Geometry: final body of the model. Coordinates: model frame, mm. Give positions to 0.01 mm unless a question says otherwise; leave off trailing zeros. Loops run counter-clockwise (first coordinate to the right, second up) from the corner with the lowest first, then second, coordinate; pieces in that order, holes last.
1. First-contact query: P1, Ø0.8, axis at y = 33.5, z = 0.5, coming from the -X side; P2, Ø0.8, axis at y = 17.5, z = 1, coming from the -X side. Flat tips, straight axial feed; report the tip coordinate or a pass-through.
2. Section A-A, the plane y = 32.5. Output: boundary loops of the cut face in (x, z), then the cut area to 3 significant figures.
3. Section C-C, the plane y = 7.1. Output: boundary loops of the cut face in (x, z), then the cut area to 3 significant figures.
4. Section D-D, the plane z = 0.9. State how many separate pieces and enclosed holes the cut face has, then the cut area to 3 significant figures.
5. Material intervals for line 1 along Y through (x, z) = (2, 0.65); line 2 along X through (y, z) = (60.5, 0.85); line 3 along Y through (x, z) = (13, 0.2), sorted ascending.
6. Section B-B, the plane x = 11.6. Output: boundary loops of the cut face in (y, z), then the cut area to 3 significant figures.
Autodesk Inventor part; units mm, degrees
ref_plane "YZ Plane" through (0, 0, 0) normal (1, 0, 0) x (0, 1, 0)
ref_plane "XZ Plane" through (0, 0, 0) normal (0, 1, 0) x (-1, 0, 0)
ref_plane "XY Plane" through (0, 0, 0) normal (0, 0, 1) x (1, 0, 0)
sketch "スケッチ1" plane through (0, 0, 0) normal (0, 0, 1) x (1, 0, 0)
  line L0 (0, 0) -> (32, 0)
  line L1 (32, 0) -> (32, 63)
  line L2 (32, 63) -> (0, 63)
  line L3 (0, 63) -> (0, 0)
  dimension "d0" = 32
  dimension "d1" = 63
extrude "押し出し1" add sketch "スケッチ1" along normal blind 1.5
sketch "スケッチ2" plane through (0, 0, 1.5) normal (0, 0, 1) x (1, 0, 0)
  line L0 (2, 60.5) -> (30, 60.5)
  line L1 (30, 60.5) -> (30, 32.5)
  line L2 (30, 32.5) -> (2, 32.5)
  line L3 (2, 32.5) -> (2, 60.5)
  line L4 (32, 63) -> (0, 63)
  line L5 (16, 63) -> (16, 60.5)
  point P0 (0, 0)
  dimension "d4" = 28
  dimension "d5" = 28
  dimension "d6" = 2.5
hole "穴1" at (30, 60.5, 1.5) at (2, 60.5, 1.5) at (30, 32.5, 1.5) at (2, 32.5, 1.5) direction (0, 0, -1) diameter 1.567 end through all
sketch "スケッチ3" plane through (0, 0, 1.5) normal (0, 0, 1) x (1, 0, 0)
  circle A0 centre (30, 32.5) radius 0.7835
  circle A1 centre (30, 60.5) radius 0.7835
  circle A2 centre (2, 60.5) radius 0.7835
  circle A3 centre (2, 32.5) radius 0.7835
  line L0 (0, 0) -> (32, 0)
  line L1 (32, 0) -> (32, 63)
  line L2 (32, 63) -> (0, 63)
  line L3 (0, 63) -> (0, 0)
  line L4 (0, 0) -> (8, 0)
  line L5 (8, 0) -> (8, 22.6)
  line L6 (8, 22.6) -> (0, 22.6)
  line L7 (0, 22.6) -> (0, 0)
  line L8 (0, 0) -> (32, 0)
  line L9 (16, 0) -> (16, 3.4564)
  line L10 (32, 0) -> (24, 0)
  line L11 (24, 0) -> (24, 22.6)
  line L12 (24, 22.6) -> (32, 22.6)
  line L13 (32, 22.6) -> (32, 0)
  dimension "d14" = 22.6
  dimension "d15" = 16
extrude "押し出し2" cut sketch "スケッチ3" against normal through all contours L3 L6 L5 L0 | L11 L12 L1 L0
sketch "スケッチ4" plane through (0, 0, 1.5) normal (0, 0, 1) x (1, 0, 0)
  line L0 (8, 22.6) -> (8, 0)
  line L1 (8, 0) -> (24, 0)
  line L2 (24, 0) -> (24, 22.6)
  line L3 (24, 22.6) -> (32, 22.6)
  line L4 (32, 22.6) -> (32, 63)
  line L5 (32, 63) -> (0, 63)
  line L6 (0, 63) -> (0, 22.6)
  line L7 (0, 22.6) -> (8, 22.6)
  circle A0 centre (30, 32.5) radius 0.7835
  circle A1 centre (30, 60.5) radius 0.7835
  circle A2 centre (2, 60.5) radius 0.7835
  circle A3 centre (2, 32.5) radius 0.7835
  line L8 (11.6, 15.9) -> (20.4, 15.9)
  line L9 (20.4, 15.9) -> (20.4, 7.1)
  line L10 (20.4, 7.1) -> (11.6, 7.1)
  line L11 (11.6, 7.1) -> (11.6, 15.9)
  line L12 (8, 0) -> (24, 0)
  line L13 (16, 0) -> (16, 7.1)
  line L14 (24, 0) -> (24, 22.6)
  line L15 (8, 0) -> (24, 0)
  point P0 (0, 0)
  dimension "d18" = 8.8
  dimension "d19" = 8.8
  dimension "d27" = 6.7
hole "穴2" at (20.4, 15.9, 1.5) at (20.4, 7.1, 1.5) at (11.6, 7.1, 1.5) at (11.6, 15.9, 1.5) direction (0, 0, -1) diameter 1.567 end through all
sketch "スケッチ5" plane through (0, 0, 0) normal (0, 0, -1) x (-1, 0, 0)
  line L0 (-6, 34.6) -> (-14, 34.6)
  line L1 (-14, 34.6) -> (-14, 31.4)
  line L2 (-14, 31.4) -> (-6, 31.4)
  line L3 (-6, 31.4) -> (-6, 34.6)
  line L4 (-14.5, 35.1) -> (-5.5, 35.1)
  line L5 (-5.5, 35.1) -> (-5.5, 30.9)
  line L6 (-5.5, 30.9) -> (-14.5, 30.9)
  line L7 (-14.5, 30.9) -> (-14.5, 35.1)
  point P0 (0, 0)
  dimension "d28" = 0.5
extrude "押し出し3" cut sketch "スケッチ5" against normal through all contours L3 L2 L1 L0 | L4 L5 L6 L7
fillet "フィレット1" radius 2 6 edges at (32, 63, 0.75) (0, 63, 0.75) (0, 22.6, 0.75) (32, 22.6, 0.75) (8, 0, 0.75) (24, 0, 0.75)
sketch "スケッチ6" plane through (0, 0, 1.5) normal (0, 0, 1) x (1, 0, 0)
  line L0 (14.5, 35.1) -> (14.5, 30.9)
  line L1 (14.5, 30.9) -> (5.5, 30.9)
  line L2 (5.5, 30.9) -> (5.5, 35.1)
  line L3 (5.5, 35.1) -> (14.5, 35.1)
  circle A0 centre (11.6, 7.1) radius 0.7835
  circle A1 centre (20.4, 15.9) radius 0.7835
  circle A2 centre (20.4, 7.1) radius 0.7835
  circle A3 centre (11.6, 15.9) radius 0.7835
  arc A4 (22, 0) -> (24, 2) centre (22, 2) ccw
  line L4 (24, 2) -> (24, 22.6)
  line L5 (24, 22.6) -> (30, 22.6)
  arc A5 (30, 22.6) -> (32, 24.6) centre (30, 24.6) ccw
  line L6 (32, 24.6) -> (32, 61)
  arc A6 (32, 61) -> (30, 63) centre (30, 61) ccw
  line L7 (30, 63) -> (2, 63)
  arc A7 (2, 63) -> (0, 61) centre (2, 61) ccw
  line L8 (0, 61) -> (0, 24.6)
  arc A8 (0, 24.6) -> (2, 22.6) centre (2, 24.6) ccw
  line L9 (2, 22.6) -> (8, 22.6)
  line L10 (8, 22.6) -> (8, 2)
  arc A9 (8, 2) -> (10, 0) centre (10, 2) ccw
  line L11 (10, 0) -> (22, 0)
  circle A10 centre (30, 32.5) radius 0.7835
  circle A11 centre (30, 60.5) radius 0.7835
  circle A12 centre (2, 60.5) radius 0.7835
  circle A13 centre (2, 32.5) radius 0.7835
  line L12 (8, 22.6) -> (2, 22.6)
  circle A14 centre (7.25, 22.6) radius 0.75
  line L13 (30, 22.6) -> (24, 22.6)
  circle A15 centre (24.75, 22.6) radius 0.75
  line L14 (8, 22.6) -> (8, 2)
  line L15 (24, 2) -> (24, 22.6)
  point P0 (0, 0)
  dimension "d34" = 1.5
  dimension "d35" = 1.5
extrude "押し出し4" cut sketch "スケッチ6" against normal through all contours A15 L5 | L5 A15 | A14 L9 | L9 A14
fillet "フィレット2" radius 1 4 edges at (8, 22.6, 0.75) (6.5, 22.6, 0.75) (25.5, 22.6, 0.75) (24, 22.6, 0.75)
sketch "スケッチ7" plane through (0, 0, 1.5) normal (0, 0, 1) x (1, 0, 0)
  arc A0 (25.3655, 23.0286) -> (26.1861, 22.6) centre (26.1861, 23.6) ccw
  line L0 (26.1861, 22.6) -> (30, 22.6)
  arc A1 (30, 22.6) -> (32, 24.6) centre (30, 24.6) ccw
  line L1 (32, 24.6) -> (32, 61)
  arc A2 (32, 61) -> (30, 63) centre (30, 61) ccw
  line L2 (30, 63) -> (2, 63)
  arc A3 (2, 63) -> (0, 61) centre (2, 61) ccw
  line L3 (0, 61) -> (0, 24.6)
  arc A4 (0, 24.6) -> (2, 22.6) centre (2, 24.6) ccw
  line L4 (2, 22.6) -> (5.8139, 22.6)
  arc A5 (5.8139, 22.6) -> (6.6345, 23.0286) centre (5.8139, 23.6) ccw
  arc A6 (8, 22.6) -> (6.6345, 23.0286) centre (7.25, 22.6) ccw
  line L5 (8, 22.6) -> (8, 2)
  arc A7 (8, 2) -> (10, 0) centre (10, 2) ccw
  line L6 (10, 0) -> (22, 0)
  arc A8 (22, 0) -> (24, 2) centre (22, 2) ccw
  line L7 (24, 2) -> (24, 22.6)
  arc A9 (25.3655, 23.0286) -> (24, 22.6) centre (24.75, 22.6) ccw
  line L8 (14.5, 35.1) -> (14.5, 30.9)
  line L9 (14.5, 30.9) -> (5.5, 30.9)
  line L10 (5.5, 30.9) -> (5.5, 35.1)
  line L11 (5.5, 35.1) -> (14.5, 35.1)
  circle A10 centre (11.6, 7.1) radius 0.7835
  circle A11 centre (20.4, 15.9) radius 0.7835
  circle A12 centre (20.4, 7.1) radius 0.7835
  circle A13 centre (11.6, 15.9) radius 0.7835
  circle A14 centre (30, 32.5) radius 0.7835
  circle A15 centre (30, 60.5) radius 0.7835
  circle A16 centre (2, 60.5) radius 0.7835
  circle A17 centre (2, 32.5) radius 0.7835
  circle A18 centre (2, 60.5) radius 0.7835
  line L12 (2, 60.5) -> (30, 60.5)
  line L13 (30, 60.5) -> (30, 32.5)
  line L14 (30, 32.5) -> (2, 32.5)
  line L15 (2, 32.5) -> (2, 60.5)
  line L16 (26.5, 57) -> (5.5, 57)
  line L17 (5.5, 57) -> (5.5, 36)
  line L18 (5.5, 36) -> (26.5, 36)
  line L19 (26.5, 36) -> (26.5, 57)
  point P0 (0, 0)
  dimension "d38" = 21
extrude "押し出し5" cut sketch "スケッチ7" against normal through all contours L19 L18 L17 L16
sketch "スケッチ8" plane through (0, 0, 1.5) normal (0, 0, 1) x (1, 0, 0)
  line L0 (5.5, 36) -> (5.5, 57)
  line L1 (5.5, 57) -> (26.5, 57)
  line L2 (26.5, 57) -> (26.5, 36)
  line L3 (26.5, 36) -> (5.5, 36)
  arc A0 (25.3655, 23.0286) -> (26.1861, 22.6) centre (26.1861, 23.6) ccw
  line L4 (26.1861, 22.6) -> (30, 22.6)
  arc A1 (30, 22.6) -> (32, 24.6) centre (30, 24.6) ccw
  line L5 (32, 24.6) -> (32, 61)
  arc A2 (32, 61) -> (30, 63) centre (30, 61) ccw
  line L6 (30, 63) -> (2, 63)
  arc A3 (2, 63) -> (0, 61) centre (2, 61) ccw
  line L7 (0, 61) -> (0, 24.6)
  arc A4 (0, 24.6) -> (2, 22.6) centre (2, 24.6) ccw
  line L8 (2, 22.6) -> (5.8139, 22.6)
  arc A5 (5.8139, 22.6) -> (6.6345, 23.0286) centre (5.8139, 23.6) ccw
  arc A6 (8, 22.6) -> (6.6345, 23.0286) centre (7.25, 22.6) ccw
  line L9 (8, 22.6) -> (8, 2)
  arc A7 (8, 2) -> (10, 0) centre (10, 2) ccw
  line L10 (10, 0) -> (22, 0)
  arc A8 (22, 0) -> (24, 2) centre (22, 2) ccw
  line L11 (24, 2) -> (24, 22.6)
  arc A9 (25.3655, 23.0286) -> (24, 22.6) centre (24.75, 22.6) ccw
  line L12 (14.5, 35.1) -> (14.5, 30.9)
  line L13 (14.5, 30.9) -> (5.5, 30.9)
  line L14 (5.5, 30.9) -> (5.5, 35.1)
  line L15 (5.5, 35.1) -> (14.5, 35.1)
  circle A10 centre (11.6, 7.1) radius 0.7835
  circle A11 centre (20.4, 15.9) radius 0.7835
  circle A12 centre (20.4, 7.1) radius 0.7835
  circle A13 centre (11.6, 15.9) radius 0.7835
  circle A14 centre (30, 32.5) radius 0.7835
  circle A15 centre (30, 60.5) radius 0.7835
  circle A16 centre (2, 60.5) radius 0.7835
  circle A17 centre (2, 32.5) radius 0.7835
  line L16 (5.5, 36) -> (5.5, 35.1)
  line L17 (14.5, 35.1) -> (14.5, 36)
  point P0 (0, 0)
extrude "押し出し6" cut sketch "スケッチ8" against normal through all contours L3 L17 L15 L16
fillet "フィレット5" radius 1 6 edges at (5.5, 57, 0.75) (26.5, 57, 0.75) (26.5, 36, 0.75) (14.5, 30.9, 0.75) (5.5, 30.9, 0.75) (14.5, 36, 0.75)
properties part number "手先カメラ" material "アルミニウム 6061"
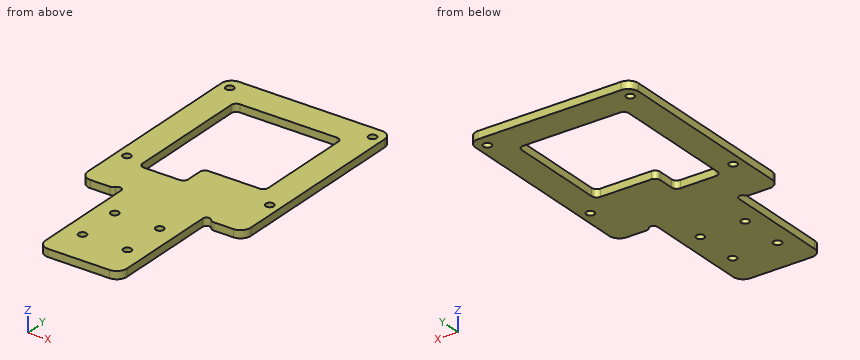
Answers below:
1. P1: stops at x = 0
1. P2: stops at x = 8
2. outline: (0, 0) - (1.22, 0) - (1.22, 1.5) - (0, 1.5) - close; (2.78, 0) - (5.5, 0) - (5.5, 1.5) - (2.78, 1.5) - close; (14.5, 0) - (29.22, 0) - (29.22, 1.5) - (14.5, 1.5) - close; (30.78, 0) - (32, 0) - (32, 1.5) - (30.78, 1.5) - close
2. area: 29.8 mm2
3. outline: (8, 0) - (10.82, 0) - (10.82, 1.5) - (8, 1.5) - close; (12.38, 0) - (19.62, 0) - (19.62, 1.5) - (12.38, 1.5) - close; (21.18, 0) - (24, 0) - (24, 1.5) - (21.18, 1.5) - close
3. area: 19.3 mm2
4. separate pieces: 1
4. enclosed holes: 9
4. area: 1,150 mm2
5. line 1: y = 22.6 to 31.72, 33.28 to 59.72, 61.28 to 63
5. line 2: x = 0 to 1.22, 2.78 to 29.22, 30.78 to 32
5. line 3: y = 0 to 30.9, 57 to 63
6. outline: (0, 0) - (6.32, 0) - (6.32, 1.5) - (0, 1.5) - close; (7.88, 0) - (15.12, 0) - (15.12, 1.5) - (7.88, 1.5) - close; (16.68, 0) - (30.9, 0) - (30.9, 1.5) - (16.68, 1.5) - close; (57, 0) - (63, 0) - (63, 1.5) - (57, 1.5) - close
6. area: 50.6 mm2
